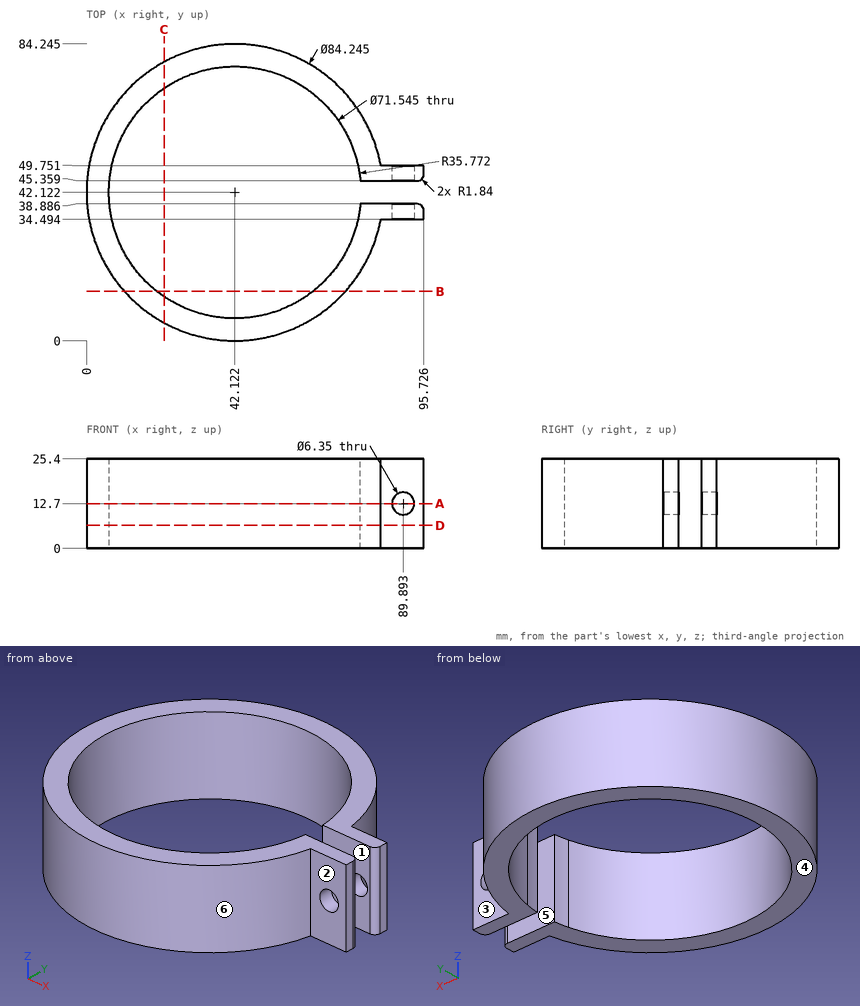
Study the drawing (mm; zero at the part's minimum x, y, z) and answer. A direction names the side the tool comes from. Coordinates: 2 decimals unless noted, no trailing zeros. Write each loop counter-clockwise with the first axis right and the second up, starting at its lowest first coordinate (ties: lowest second). Pieces come first, ordered by that corner, then holes. Notation, with made-up numbers: (42, -12) - (99, -12) arc R20 cw to (99, 19) - close; hole circle Ø10 at (-7.5, 52). An arc over 180 degrees is marked (long way). One line per item, written item: value.
1) Each of these flat-tipped pins is pushed along its axis until it touches: pin 1 Ø6 at (x, z) = (55.5, 4) entering from +Y; pin 2 Ø13 at (x, z) = (82, 19) entering from -Y; pin 3 Ø5 at (x, z) = (89.89, 12.7) entering from -Y; pin 4 Ø13 at (x, z) = (87, 13.5) entering from +Y (1 decimal). Where does it stop, or does it pass through?
Geometry check:
pin 1: stops at y = 82.95
pin 2: stops at y = 16.43
pin 3: passes through
pin 4: stops at y = 59.5
2) For a pull along Y with two mould halves and no side action, classify the marked faces 4, 5 and 6 as pulls with the +Y half, pulls with the -Y half, needs draft (parallel to the pull), parting line crosses it, or undercut.
Geometry check:
face 4: needs draft
face 5: undercut
face 6: parting line crosses it
3) Find section D-D (z = 6.5). Give the vertices of the cut face in (x, y) (1 decimal).
Geometry check:
outline: (77.1, 34.5) arc R35.8 cw (long way) to (77.1, 49.8) arc R35.8 cw to (77.7, 45.4) - (93.9, 45.4) arc R1.8 ccw to (95.7, 47.2) - (95.7, 49.8) - (83.5, 49.8) arc R42.1 ccw (long way) to (83.5, 34.5) - (95.7, 34.5) - (95.7, 37) arc R1.8 ccw to (93.9, 38.9) - (77.7, 38.9) arc R35.8 cw to start
4) Consider line 1 along X through (y, z) = (37, 11) (1 decimal); line 2 along Y through (x, z) = (41, 21.5) (1 decimal); line 3 along Y through (x, z) = (84, 1.5) (1 decimal). Determine where each line is inside the solid, lowest interval first. Write a range as from..to.
Geometry check:
line 1: x = 0.3..6.7, 77.5..87.2, 92.6..95.7
line 2: y = 0..6.4, 77.9..84.2
line 3: y = 34.5..38.9, 45.4..49.8
5) Find section C-C (x = 22). Give the vertices of the cut face in (y, z).
Geometry check:
outline: (5.12, 0) - (12.55, 0) - (12.55, 25.4) - (5.12, 25.4) - close; (71.7, 0) - (79.13, 0) - (79.13, 25.4) - (71.7, 25.4) - close
6) Find section A-A (z = 12.7). Give the vertices of the cut face in (x, y) (1 decimal), and give its area (3 significant figures).
Geometry check:
outline: (77.1, 34.5) arc R35.8 cw (long way) to (77.1, 49.8) arc R35.8 cw to (77.7, 45.4) - (86.7, 45.4) - (86.7, 49.8) - (83.5, 49.8) arc R42.1 ccw (long way) to (83.5, 34.5) - (86.7, 34.5) - (86.7, 38.9) - (77.7, 38.9) arc R35.8 cw to start; (93.1, 34.5) - (95.7, 34.5) - (95.7, 37) arc R1.8 ccw to (93.9, 38.9) - (93.1, 38.9) - close; (93.1, 45.4) - (93.9, 45.4) arc R1.8 ccw to (95.7, 47.2) - (95.7, 49.8) - (93.1, 49.8) - close
area: 1,560 mm2
7) Find section B-B (y = 14). Give the vertices of the cut face in (x, z).
Geometry check:
outline: (10.76, 0) - (20.01, 0) - (20.01, 25.4) - (10.76, 25.4) - close; (64.23, 0) - (73.48, 0) - (73.48, 25.4) - (64.23, 25.4) - close
8) A tool of negligible diameter and unlimited length cuts with its end or side. For the marked faces 1, 2 and 3, from which of +Z, -Z, +X, -X, +Y, -Y can it reach the whole face along a straight path? Write none if from no direction.
Geometry check:
face 1: +Z, -Z, +X
face 2: +Z, -Z, +X, -Y
face 3: +Z, -Z, +X, +Y
